```python
from build123d import *

# Parameters (mm, degrees)
SKETCH2_W           = 430
SKETCH2_H           = 420
SKETCH2_R           = 2.6
BOSS_EXTRUDE1_DEPTH = 3.175
CHAMFER1_SIZE       = 3


with BuildPart() as part:
    # Sketch2 → Boss-Extrude1 (new body, symmetric)
    with BuildSketch(Plane(origin=(0, 0, 0), x_dir=(1, 0, 0), z_dir=(0, 1, 0))):
        Rectangle(SKETCH2_W, SKETCH2_H)
        with Locations((-205, 200)):
            Circle(SKETCH2_R, mode=Mode.SUBTRACT)
        with Locations((205, 200)):
            Circle(SKETCH2_R, mode=Mode.SUBTRACT)
        with Locations((205, -200)):
            Circle(SKETCH2_R, mode=Mode.SUBTRACT)
        with Locations((-205, -200)):
            Circle(SKETCH2_R, mode=Mode.SUBTRACT)
        with Locations((-205, 0)):
            Circle(SKETCH2_R, mode=Mode.SUBTRACT)
        with Locations((205, 0)):
            Circle(SKETCH2_R, mode=Mode.SUBTRACT)
    extrude(amount=BOSS_EXTRUDE1_DEPTH, both=True)

    # Chamfer1
    chamfer1_edges = [part.edges().sort_by_distance(p)[0] for p in [
        (-207.6, 3.175, -200),
        (202.4, 3.175, -200),
        (202.4, 3.175, 200),
        (-207.6, 3.175, 200),
        (-207.6, 3.175, 0),
        (202.4, 3.175, 0),
    ]]
    chamfer(chamfer1_edges, length=CHAMFER1_SIZE)


solid = part.part
```
The model under review builds one solid part; all positions refer to its coordinate system, in mm. Give positions to 0.01 mm unless a question says otherwise; leave off trailing zeros. Answer in a Markdown table with one row per item.
1) Mouldability with a two-part tool opening along X and no side actions: class faces 1 (the conical face through (207.536, 0.321, -198.948)), 2 (the flat face through (-3, 3.175, -3)) as +X half, -X half, draft (parallel to the pull), parting line (faces both ways), or undercut.
Worked answers:
| item | result |
|---|---|
| face 1 | undercut |
| face 2 | draft |
2) Clearance check with a flat-ended pin moving along its axis: P1, Ø6, axis at x = 205, z = 0, coming from the -Y side (3 decimals). State where the tip first meets the part, or that it passes through.
Worked answers:
| item | result |
|---|---|
| P1 | y = -3.175 |
3) For L1, parallel to Z at x = -205, y = -1.25; L2, parallel to X at y = -0.85, z = 0; L3, parallel to X at y = 1.75, z = -3, list the stretches that pass through material, from the lowest coordinate up. Write a range as [from, to].
Worked answers:
| item | result |
|---|---|
| L1 | [-210, -202.6], [-197.4, -2.6], [2.6, 197.4], [202.6, 210] |
| L2 | [-215, -207.6], [-202.4, 202.4], [207.6, 215] |
| L3 | [-215, -207.9], [-202.1, 202.1], [207.9, 215] |
